Input: dimensioned drawing with shaded views. Units: mm. Origin: part minimum x, y, z. Give positions to 0.01 mm unless a question says otherwise; leave off trailing zeros. Loops run counter-clockwise (first coordinate to the right, second up) from the corner with the lowest first, then second, coordinate; pieces in that order, holes last. Notation, with made-up numbers: (-20, -37) -> (-9, -37) arc R20 ccw to (-9, -28) -> close; hole circle Ø1 at (-12.5, -27). An arc over 180 degrees is marked (long way). Answer in a Markdown table with one row per item. Add a question column.
1) Section query C-C (x = 19.25). Return the cut outline in (y, z).
2) Draft query along X for the marked faces 1, 2 and 3. Return one class per face: +X half, -X half, draft (parallel to the pull), parting line (faces both ways), or undercut.
3) First-contact query: P1, Ø9, axis at x = 15, z = 15, coming from the +Y side; P2, Ø3, axis at y = 28.5, z = 13.5, coming from the +X side; P3, Ø12, axis at y = 34.5, z = 19, coming from the -X side; P4, Ø3, axis at x = 13, y = 48, coming from the -Z side. Flat tips, straight axial feed; report the tip coordinate or a pass-through.
4) Line query: line 1 (Z direction, x = 15, y = 45); line 2 (Y direction, x = 8.5, z = 18); line 3 (Z direction, x = 17.25, y = 39.5). Output: solid intervals per line, ascending. Write a range as from..to.
5) Section query D-D (y = 37). Return the cut outline in (x, z), plus the area to 3 significant figures.
6) Section query A-A (z = 15). Return the cut outline in (x, y).
7) Section query B-B (x = 15). Return the cut outline in (y, z).
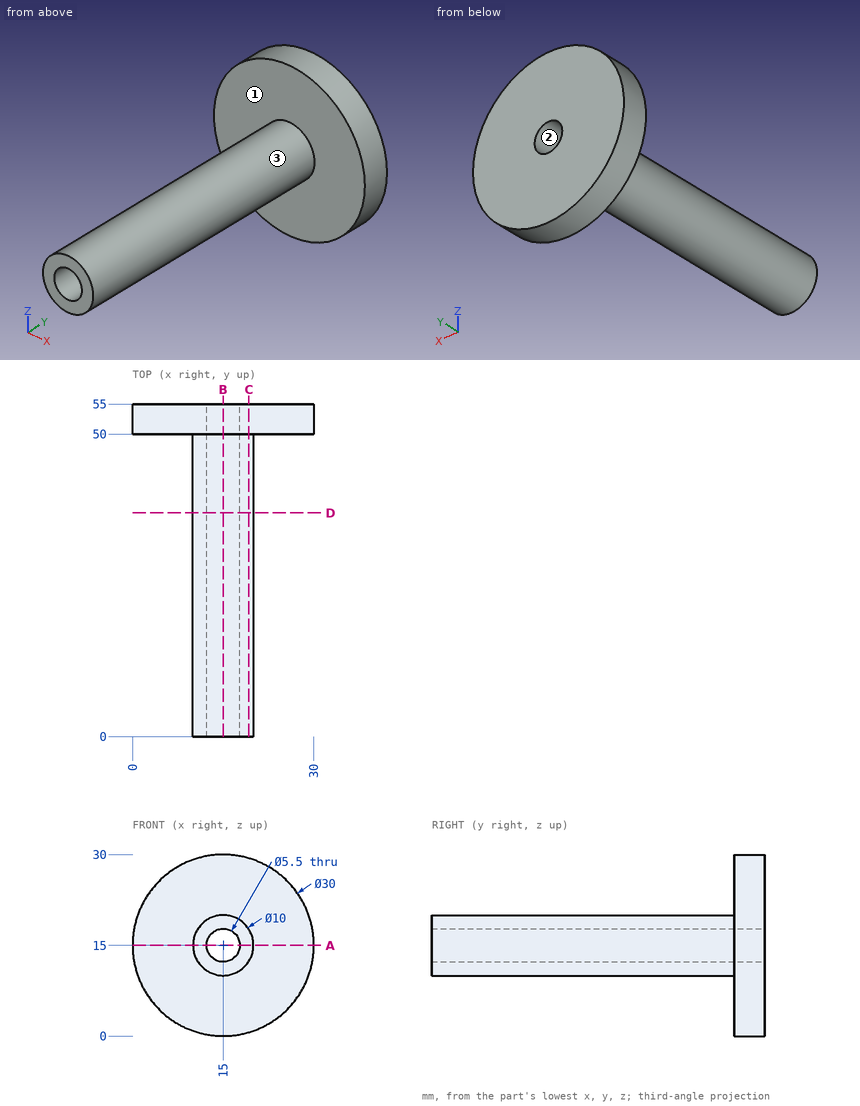
Evaluation:
| question | item | result |
|---|---|---|
| 1 | outline | (0, 12.37) -> (50, 12.37) -> (50, 0.61) -> (55, 0.61) -> (55, 29.39) -> (50, 29.39) -> (50, 17.63) -> (0, 17.63) -> close |
| 2 | face 1 | draft |
| 2 | face 2 | undercut |
| 2 | face 3 | parting line |
| 3 | P1 | y = 55 |
| 3 | P2 | x = 20 |
| 3 | P3 | x = 10 |
| 3 | P4 | z = 10.03 |
| 4 | line 1 | 10..12.25, 17.75..20 |
| 4 | line 2 | 50..55 |
| 4 | line 3 | 10.53..13.42, 16.58..19.47 |
| 5 | outline | circle Ø10 at (15, 15); hole circle Ø5.5 at (15, 15) |
| 5 | area | 54.8 mm² |
| 6 | outline | (0, 50) -> (10, 50) -> (10, 0) -> (12.25, 0) -> (12.25, 55) -> (0, 55) -> close; (17.75, 0) -> (20, 0) -> (20, 50) -> (30, 50) -> (30, 55) -> (17.75, 55) -> close |
| 7 | outline | (0, 10) -> (50, 10) -> (50, 0) -> (55, 0) -> (55, 12.25) -> (0, 12.25) -> close; (0, 17.75) -> (55, 17.75) -> (55, 30) -> (50, 30) -> (50, 20) -> (0, 20) -> close |
